from build123d import *

# Parameters (mm, degrees)
SKETCH1_W           = 12
SKETCH1_H           = 88
SKETCH1_R           = 1.5
BOSS_EXTRUDE1_DEPTH = 2
SKETCH2_W           = 12
SKETCH2_H           = 2
BOSS_EXTRUDE2_DEPTH = 135
FILLET1_R           = 8
SKETCH3_R           = 1.939400698
CUT_EXTRUDE1_DEPTH  = 163.065945849


with BuildPart() as part:
    # Sketch1 → Boss-Extrude1 (new body)
    with BuildSketch(Plane.XY):
        with Locations((6, 44)):
            Rectangle(SKETCH1_W, SKETCH1_H)
        with Locations((6, 82)):
            Circle(SKETCH1_R, mode=Mode.SUBTRACT)
        with Locations((6, 23)):
            Circle(SKETCH1_R, mode=Mode.SUBTRACT)
    extrude(amount=BOSS_EXTRUDE1_DEPTH)

    # Sketch2 → Boss-Extrude2 (add)
    with BuildSketch(Plane.XY.offset(2)):
        with Locations((6, 1)):
            Rectangle(SKETCH2_W, SKETCH2_H)
    extrude(amount=BOSS_EXTRUDE2_DEPTH)

    # Fillet1
    # the kernel refuses this fillet: 8 mm, written as the material it takes off along each edge
    with BuildSketch(Plane(origin=(12, 88, -20), x_dir=(-1, 0, 0), z_dir=(0, 0, 1))) as fillet1_piece_1:
        with BuildLine():
            CenterArc((FILLET1_R, FILLET1_R), FILLET1_R, 180, 90)
            Line((0, FILLET1_R), (0, 0))
            Line((0, 0), (FILLET1_R, 0))
        make_face()
    extrude(amount=42, mode=Mode.SUBTRACT)
    with BuildSketch(Plane(origin=(0, 88, -20), x_dir=(1, 0, 0), z_dir=(0, 0, 1))) as fillet1_piece_2:
        with BuildLine():
            CenterArc((FILLET1_R, -FILLET1_R), FILLET1_R, 90, 90)
            Line((0, -FILLET1_R), (0, 0))
            Line((0, 0), (FILLET1_R, 0))
        make_face()
    extrude(amount=42, mode=Mode.SUBTRACT)

    # Sketch3 → Cut-Extrude1 (cut, through all)
    with BuildSketch(Plane(origin=(0, 2, 0), x_dir=(1, 0, 0), z_dir=(0, 1, 0))):
        with Locations(Location((6, -131, 0), (0, 0, 270))):
            Circle(SKETCH3_R)
        with Locations(Location((6, -8, 0), (0, 0, 270))):
            Circle(SKETCH3_R)
    extrude(amount=-CUT_EXTRUDE1_DEPTH, mode=Mode.SUBTRACT)


solid = part.part
Source: CAD feature listing. Evaluate the final solid. Frame: model axes, mm. A direction names the side the tool comes from. Coordinates: 2 decimals unless noted, no trailing zeros. Loops run counter-clockwise (first coordinate to the right, second up) from the corner with the lowest first, then second, coordinate; pieces in that order, holes last. Notation, with made-up numbers: (24.5, 83.25) - (37.5, 83.25) arc R30 ccw to (37.5, 115.25) - close; hole circle Ø2 at (43, 19.25). An arc over 180 degrees is marked (long way). One line per question, with ' | ' between items.
1) Section A-A, the plane z = 131. Return loops of the section in (x, y).
Report:
outline: (0, 0) - (4.06, 0) - (4.06, 2) - (0, 2) - close; (7.94, 0) - (12, 0) - (12, 2) - (7.94, 2) - close
2) Pull-direction query (X, two-part tool) for faces 1 (the face through (10.4, 84.8, 1)), 2 (the face through (6, 0, 68)), 3 (the face through (6.58, 1.01, 132.85)); classes: released by +X, released by -X, zero draft, split by the parting line, or undercut.
Report:
face 1: released by +X | face 2: zero draft | face 3: undercut
3) Set-up query: faces 4 (the face through (6, 45, 2)), 5 (the face through (5.805, 83.487, 0.986)). Return all of +Z, -Z, +X, -X, +Y, -Y with unobstructed straight access to the full face (end or side cutting, diameter ignored); none if empty.
Report:
face 4: +Z, +X, -X, +Y | face 5: +Z, -Z
4) Line query: line 1 along Y through (x, z) = (6, 1.1); line 2 along X through (y, z) = (1.15, 131); line 3 along Z through (x, y) = (10.25, 65). Output: solid intervals per line, ascending.
Report:
line 1: y = 0 to 21.5, 24.5 to 80.5, 83.5 to 87.75 | line 2: x = 0 to 4.06, 7.94 to 12 | line 3: z = 0 to 2
5) Section C-C, the plane z = 16. Return loops of the section in (x, y), then the cut area to 3 significant figures.
Report:
outline: (0, 0) - (12, 0) - (12, 2) - (0, 2) - close | area: 24.0 mm²
6) Section B-B, the plane y = 23. Return loops of the section in (x, z).
Report:
outline: (0, 0) - (4.5, 0) - (4.5, 2) - (0, 2) - close; (7.5, 0) - (12, 0) - (12, 2) - (7.5, 2) - close
7) First-contact query: P1, Ø1.5, axis at x = 2.5, y = 12, coming from the +Z side; P2, Ø2, axis at x = 7.5, z = 51.5, coming from the -Y side; P3, Ø2.5, axis at x = 6, y = 82, coming from the +Z side; P4, Ø1.5, axis at x = 3.5, z = 50, coming from the +Y side. Flat tips, straight axial feed; report the tip coordinate or a pass-through.
Report:
P1: stops at z = 2 | P2: stops at y = 0 | P3: passes through | P4: stops at y = 2
